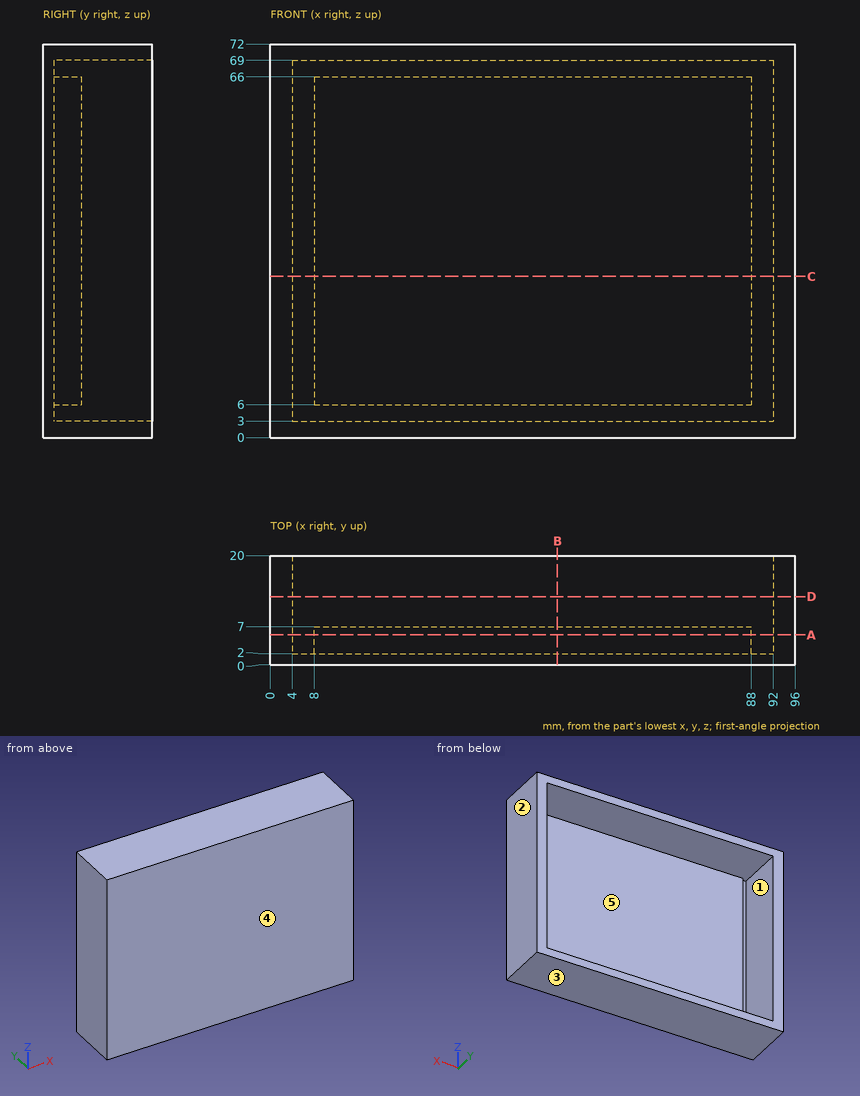
The figure shows three views and two pictorial views of one solid part (mm, origin at its lowest corner). Answer the questions. A direction names the side the tool comes from. Give positions to 0.01 mm unless a question says otherwise; leave off trailing zeros. Write each loop counter-clockwise with the first axis right and the second up, starting at its lowest first coordinate (ties: lowest second). Pieces come first, ordered by that corner, then holes. Notation, with made-up numbers: M 59,-11 L 66,-11 A15 ccw 66,18 Z; hole C 41.25,80 d10. An arc over 180 degrees is marked long. One line per item, written item: value. Start each with the question number.
(1) Find section D-D (y = 12.5). Determine the outline of the cut face in (x, z).
(2) Find section B-B (x = 52.5). Determine the outline of the cut face in (y, z), plus the area to 3 significant figures.
(3) Determine the mould class of the marked faces 1, 2 and 3 for opening direction Z: pulls with the +Z half, pulls with the -Z half, needs draft (parallel to the pull), parting line crosses it, or undercut.
(4) Find section C-C (z = 29.5). Determine the outline of the cut face in (x, y).
(5) A flat-ended cylindrical pin translates along its axis: pin 1 Ø1 at (x, z) = (41, 19) entering from +Y. Find the tip coordinate at first contact, or state that the pin passes through.
(6) Find the intervals of material crossed by line 1 (X direction, y = 3, z = 10.5); line 2 (Z direction, x = 46, y = 5); line 3 (X direction, y = 9, z = 66.5), in increasing order.
(7) A tool of negligible diameter and unlimited length cuts with its end or side. For the marked faces 4 and 5, from which of +Z, -Z, +X, -X, +Y, -Y can it reach the whole face along a straight path? Write none if from no direction.
(8) Find section A-A (y = 5.5). Determine the outline of the cut face in (x, z), plus the area to 3 significant figures.
Results below:
1. outline: M 0,0 L 96,0 L 96,72 L 0,72 Z; hole M 4,3 L 92,3 L 92,69 L 4,69 Z
2. outline: M 0,0 L 20,0 L 20,3 L 2,3 L 2,6 L 7,6 L 7,66 L 2,66 L 2,69 L 20,69 L 20,72 L 0,72 Z
2. area: 552 mm^2
3. face 1: undercut
3. face 2: needs draft
3. face 3: pulls with the -Z half
4. outline: M 0,0 L 96,0 L 96,20 L 92,20 L 92,2 L 88,2 L 88,7 L 8,7 L 8,2 L 4,2 L 4,20 L 0,20 Z
5. pin 1: stops at y = 7
6. line 1: x = 0 to 4, 8 to 88, 92 to 96
6. line 2: z = 0 to 3, 6 to 66, 69 to 72
6. line 3: x = 0 to 4, 92 to 96
7. face 4: +Z, -Z, +X, -X, -Y
7. face 5: +Y
8. outline: M 0,0 L 96,0 L 96,72 L 0,72 Z; M 8,6 L 88,6 L 88,66 L 8,66 Z; hole M 4,3 L 92,3 L 92,69 L 4,69 Z
8. area: 5,900 mm^2
